Source: three-view drawing plus pictorial views. Frame: mm from the lowest corner of the part. A direction names the side the tool comes from. Give positions to 0.01 mm unless a question says otherwise; leave off trailing zeros. Write each loop counter-clockwise with the first axis right and the second up, starting at its lowest first coordinate (ties: lowest second). Pieces come first, ordered by that corner, then holes. Notation, with made-up numbers: (-1.75, 83.25) - (39.25, 83.25) arc R33 cw to (39.25, 120.25) - close; hole circle Ø9 at (80, 61.25). An arc over 180 degrees is marked (long way). One line per question, with ' | ' between items. Start each with the question number.
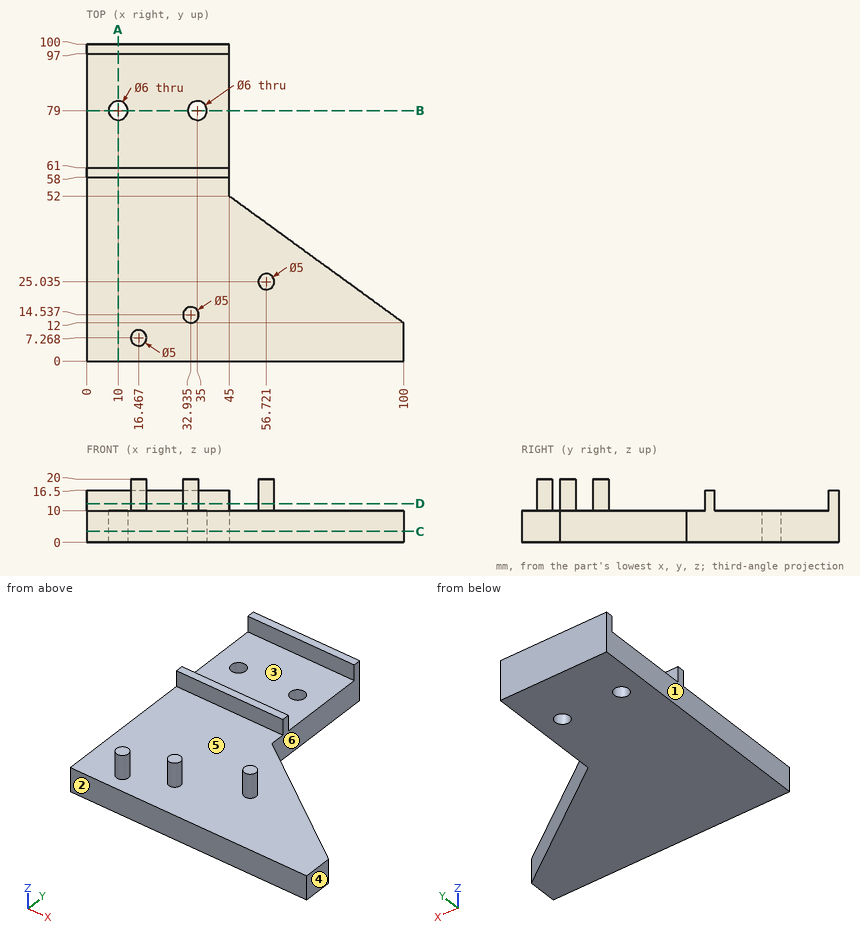
1) First-contact query: pin 1 Ø3 at (x, z) = (24.5, 14) entering from -Y; pin 2 Ø0.9 at (x, y) = (13, 98) entering from +Z; pin 3 Ø4 at (x, y) = (26, 70) entering from +Z. Flat tips, straight axial feed; report the tip coordinate or a pass-through.
2) Section B-B, the plane y = 79. Output: boundary loops of the cut face in (x, z).
3) Section D-D, the plane z = 12.25. Output: boundary loops of the cut face in (x, y) (1 decimal).
4) Section C-C, the plane z = 3.5. Output: boundary loops of the cut face in (x, y).
5) Reachability of the marked faces 4, 5 and 6 from +Z, -Z, +X, -X, +Y, -Y: full face, straight path, thin tool, end or side. Return the list, or none.
6) Section A-A, the plane x = 10. Output: boundary loops of the cut face in (y, z).
7) Line query: L1, parallel to Y at x = 10, z = 3.5; L2, parallel to Y at x = 13, z = 15.5; L3, parallel to Z at x = 16.5, y = 57. Output: solid intervals per line, ascending.
8) Pull-direction query (Y, two-part tool) for the marked faces 1, 2 and 3; classes: +Y half, -Y half, draft (parallel to the pull), parting line (faces both ways), or undercut.
Answer key:
1) pin 1: y = 58 | pin 2: z = 16.5 | pin 3: z = 10
2) outline: (0, 0) - (7, 0) - (7, 10) - (0, 10) - close; (13, 0) - (32, 0) - (32, 10) - (13, 10) - close; (38, 0) - (45, 0) - (45, 10) - (38, 10) - close
3) outline: (0, 58) - (45, 58) - (45, 61) - (0, 61) - close; (0, 97) - (45, 97) - (45, 100) - (0, 100) - close; circle Ø5 at (16.5, 7.3); circle Ø5 at (32.9, 14.5); circle Ø5 at (56.7, 25)
4) outline: (0, 0) - (100, 0) - (100, 12) - (45, 52) - (45, 100) - (0, 100) - close; hole circle Ø6 at (10, 79); hole circle Ø6 at (35, 79)
5) face 4: +Z, -Z, +X, +Y, -Y | face 5: +Z | face 6: +Z, -Z, +X, +Y
6) outline: (0, 0) - (76, 0) - (76, 10) - (61, 10) - (61, 16.5) - (58, 16.5) - (58, 10) - (0, 10) - close; (82, 0) - (100, 0) - (100, 16.5) - (97, 16.5) - (97, 10) - (82, 10) - close
7) L1: 0 to 76, 82 to 100 | L2: 58 to 61, 97 to 100 | L3: 0 to 10
8) face 1: draft | face 2: -Y half | face 3: undercut
